Autodesk Inventor part; units mm, degrees
ref_plane "Work Plane2" through (0, 7.5, 40) normal (0, 1, 0) x (-1, 0, 0)
ref_plane "Work Plane4" through (7.5, 0, 130) normal (1, 0, 0) x (0, 1, 0)
ref_plane "XY Plane" through (0, 0, 0) normal (0, 0, 1) x (1, 0, 0)
sketch "Sketch1" plane through (0, 0, 0) normal (0, 0, 1) x (1, 0, 0)
  circle A0 centre (0, 0) radius 5
  dimension "d0" = 10
extrude "Extrusion1" add sketch "Sketch1" along normal blind 40
sketch "Sketch3" plane through (0, 0, 40) normal (0, 0, 1) x (1, 0, 0)
  circle A0 centre (0, 0) radius 7.5
  dimension "d13" = 15
extrude "Extrusion3" add sketch "Sketch3" along normal blind 95
sketch "Sketch4" plane through (0, 0, 135) normal (0, 0, 1) x (1, 0, 0)
  circle A0 centre (0, 0) radius 4.45
  dimension "d16" = 8.9
extrude "Extrusion4" cut sketch "Sketch4" against normal blind 55
ref_plane "Work Plane2" through (0, 7.5, 40) normal (0, 1, 0) x (-1, 0, 0)
sketch "Sketch5" plane through (0, 7.5, 40) normal (0, 1, 0) x (-1, 0, 0)
  line L0 (2.5, 95) -> (-2.5, 95)
  line L1 (-2.5, 95) -> (-2.5, 45)
  line L2 (-2.5, 45) -> (2.5, 45)
  line L3 (2.5, 45) -> (2.5, 95)
  line L4 (7.5, 95) -> (-7.5, 95)
  point P0 (0, -40)
  dimension "d19" = 0
  dimension "d20" = 5
  dimension "d21" = 2.5
  dimension "d22" = 50
extrude "Extrusion5" cut sketch "Sketch5" against normal through all
sketch "Sketch6" plane through (0, 0, 80) normal (0, 0, 1) x (1, 0, 0)
  circle A0 centre (0, 0) radius 3.2
  dimension "d25" = 6.4
extrude "Extrusion6" cut sketch "Sketch6" against normal blind 35
sketch "Sketch7" plane through (0, 0, 135) normal (0, 0, 1) x (1, 0, 0)
  line L0 (-5, 5) -> (5, 5)
  line L1 (5, 5) -> (5, -5)
  line L2 (5, -5) -> (-5, -5)
  line L3 (-5, -5) -> (-5, 5)
  circle A0 centre (0, 0) radius 3.2
  dimension "d29" = 10
  dimension "d30" = 10
  dimension "d31" = 5
  dimension "d32" = 5
extrude "Extrusion7" cut sketch "Sketch7" against normal blind 10
sketch "Sketch9" plane through (0, 0, 135) normal (0, 0, 1) x (1, 0, 0)
  circle A0 centre (0, 0) radius 10
  circle A1 centre (0, 0) radius 7.5
  dimension "d39" = 20
  dimension "d42" = 15
extrude "Extrusion8" add sketch "Sketch9" against normal blind 10
sketch "Sketch10" plane through (0, 0, 0) normal (1, 0, 0) x (0, 1, 0)
  line L0 (7.5, 132) -> (10, 132)
  line L1 (10, 132) -> (10, 128)
  line L2 (10, 128) -> (7.5, 128)
  line L3 (7.5, 128) -> (7.5, 132)
  line L4 (-10, 125) -> (10, 125)
  line L5 (0, -27) -> (0, 162)
  line L6 (10, 135) -> (10, 125)
  line L7 (9, 127.5) -> (10, 127.5)
  line L8 (10, 127.5) -> (10, 132.5)
  line L9 (10, 132.5) -> (9, 132.5)
  line L10 (9, 132.5) -> (9, 127.5)
  line L11 (-10, 135) -> (10, 135)
  point P0 (0, 0)
  dimension "d43" = 4
  dimension "d44" = 3
  dimension "d46" = 2.5
  dimension "d47" = 10
  dimension "d49" = 5
  dimension "d50" = 2.5
  dimension "d51" = 1
revolve "Revolution1" cut sketch "Sketch10" angle 360 about axis through (0, 0, -10) along (0, 0, 1) contours L0 L10 L2 L3 | L10 L9 L6 L0 | L0 L1 L2 L10 | L2 L6 L7 L10
ref_plane "Work Plane4" through (7.5, 0, 130) normal (1, 0, 0) x (0, 1, 0)
sketch "Sketch12" plane through (7.5, 0, 130) normal (1, 0, 0) x (0, 1, 0)
  circle A0 centre (0, 0) radius 0.8
  point P0 (0, -130)
  dimension "d53" = 1.6
extrude "Extrusion9" cut sketch "Sketch12" against normal through all
equation "\"d31\" = 0.5 * d30"
equation "\"d32\" = 0.5 * d29"
properties part number "Handle"
Work out the finished part from the listing and answer in its coordinate system (mm). A direction names the side the tool comes from. Give positions to 0.01 mm unless a question says otherwise; leave off trailing zeros. Loops run counter-clockwise (first coordinate to the right, second up) from the corner with the lowest first, then second, coordinate; pieces in that order, holes last. Notation, with made-up numbers: (14, 23.5) -> (57, 23.5) arc R20 cw to (57, 33.5) -> close; hole circle Ø4 at (64.25, -18). An arc over 180 degrees is marked (long way). One line per question, with ' | ' between items. Start each with the question number.
1) Section A-A, the plane z = 109 is taken. Determine the outline of the cut face in (x, y).
2) For faces 1 (the face through (-2, -9, 132.5)), 2 (the face through (0, -7.5, 126.5)), 3 (the face through (-7.5, 0.1, 128.7)), determine the directions among +Z, -Z, +X, -X, +Y, -Y from which every point of the face is accessible in a straight line to the end or side of a thin tool.
3) Section B-B, the plane x = 0 is taken. State how many separate pieces and enclosed holes the cut face has, then the cut area to 4 significant figures.
4) Determine the mould class of faces 4 (the face through (7.5, -0.1, 128.7)), 5 (the face through (7, 0, 135)), 6 (the face through (-4, -5, 130)) for opening direction Z: +Z half, -Z half, draft (parallel to the pull), parting line (faces both ways), or undercut.
5) Each of these flat-tipped pins is pushed along its axis until it touches: pin 1 (4.5 mm diameter, centred on x = 0.5, y = 0, fed in from +Z); pin 2 (1 mm diameter, centred on x = -4.5, y = 4.5, fed in from -Z); pin 3 (10 mm diameter, centred on y = -1.5, z = 104, fed in from -X). Where does it stop, or does it pass through?
6) Straight lines are drawn through the part: L1, parallel to Z at x = -4, y = -7.5; L2, parallel to Y at x = 0, z = 69.5; L3, parallel to X at y = 0, z = 87.5. For each, find the intervals that lie inside material, in ascending order.
7) Section C-C, the plane z = 20 is taken. Determine the outline of the cut face in (x, y), then the cut area to 3 significant figures.
Resolved:
1) outline: (-2.5, -7.07) -> (-2.5, -3.68) arc R4.45 cw to (-2.5, 3.68) -> (-2.5, 7.07) arc R7.5 ccw to start; (2.5, -7.07) arc R7.5 ccw to (2.5, 7.07) -> (2.5, 3.68) arc R4.45 cw to (2.5, -3.68) -> close
2) face 1: none | face 2: +Z | face 3: -X
3) separate pieces: 5 | enclosed holes: 0 | area: 834.5 mm2
4) face 4: undercut | face 5: +Z half | face 6: draft
5) pin 1: z = 45 | pin 2: z = 40 | pin 3: x = -7.5
6) L1: 125 to 128, 132 to 135 | L2: -7.5 to -3.2, 3.2 to 7.5 | L3: -7.5 to -4.45, 4.45 to 7.5
7) outline: circle Ø10 at (0, 0) | area: 78.5 mm2
